The listing builds one solid part. Answer for the finished solid, in the listing's coordinates (mm). Face numbers are marked on the shaded views. Give positions to 0.01 mm unless a question says otherwise; leave off trailing zeros. Order: outer loops, then holes, each group sorted by start corner. A loop starts at its lowest first (then second) coordinate and runs counter-clockwise, first axis right, second up. Notation, with made-up numbers: M -25.75,-12.75 L -9.75,-12.75 A16 cw -9.75,-3.75 Z; hole C 59,73 d2. An arc over 180 degrees is marked long. Answer as a JSON object with one key per item and string values. Group by question number.
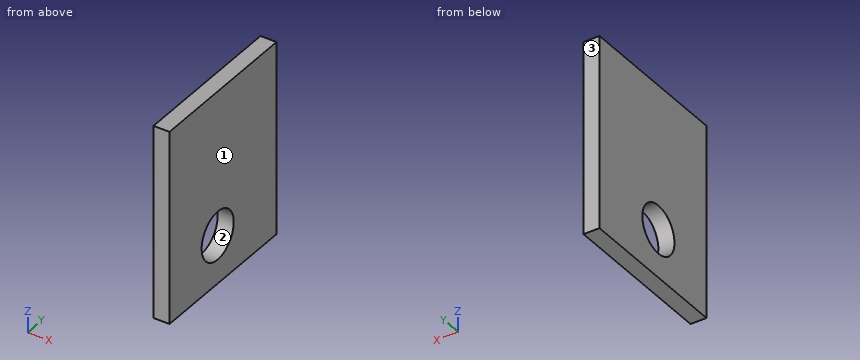
```python
from build123d import *

# Parameters (mm, degrees)
CYLINDER3125_R               = 1.5
CYLINDER3125_DEPTH           = 12
CYLINDER3127_R               = 1.5
CYLINDER3127_DEPTH           = 4
BOX1135_W                    = 6
BOX1135_H                    = 6
BOX1135_DEPTH                = 2
COMPOUND1374_PLACEMENT_ANGLE = 90
BOX1136_W                    = 1
BOX1136_H                    = 10
BOX1136_DEPTH                = 12


with BuildPart() as obj1:
    # Cylinder3125 → Cylinder3125 (new body)
    with BuildSketch(Plane(origin=(1, 14, 6), x_dir=(1, 0, 0), z_dir=(0, 0, 1))):
        Circle(CYLINDER3125_R)
    extrude(amount=CYLINDER3125_DEPTH)


with BuildPart() as obj2:
    # Cylinder3127 → Cylinder3127 (new body)
    with BuildSketch(Plane(origin=(1, 14, -0.1), x_dir=(1, 0, 0), z_dir=(0, 0, 1))):
        Circle(CYLINDER3127_R)
    extrude(amount=CYLINDER3127_DEPTH)


with BuildPart() as compound1374:
    # Box1135 → Box1135 (new body)
    with BuildSketch(Plane(origin=(-2, 11, 4), x_dir=(1, 0, 0), z_dir=(0, 0, 1))):
        with Locations((3, 3)):
            Rectangle(BOX1135_W, BOX1135_H)
    extrude(amount=BOX1135_DEPTH)

    # Compound1374: union obj1, obj2
    add(obj1.part)
    add(obj2.part)


with BuildPart() as compound1374_1:
    # Compound1374 placement: moved
    add(compound1374.part.moved(Location((6, -14, 2))).rotate(Axis((6, -14, 2), (0, 1, 0)), COMPOUND1374_PLACEMENT_ANGLE))


with BuildPart() as cut1267:
    # Box1136 → Box1136 (new body)
    with BuildSketch(Plane(origin=(21.4, -4.5, -2), x_dir=(1, 0, 0), z_dir=(0, 0, 1))):
        with Locations((0.5, 5)):
            Rectangle(BOX1136_W, BOX1136_H)
    extrude(amount=BOX1136_DEPTH)

    # Cut1267: cut Compound1374
    add(compound1374_1.part, mode=Mode.SUBTRACT)


with BuildPart() as cut1267_1:
    # Cut1267 placement: moved
    add(cut1267.part.moved(Location((0.2, 0, 0))))


solid = cut1267_1.part
```
Item 1: Determine the mould class of the marked faces 1, 2 and 3 for opening direction Y: released by +Y, released by -Y, zero draft, split by the parting line, or undercut.
Item 2: Section A-A (y = 0) is taken. Determine the outline of the cut face in (x, z), and give its area (3 significant figures).
Item 3: Section B-B (x = 22.15) is taken. Determine the outline of the cut face in (y, z).
Item 4: Consider probe 1 along Z at (x, y) = (22.05, 0); probe 2 along Y at (x, z) = (22.1, 1); probe 3 along Y at (x, z) = (21.7, 1.5). Determine where each line is inside the solid, lowest interval first. Write a range as from..to.
Item 5: Section C-C (z = 1) is taken. Determine the outline of the cut face in (x, y).
Values found:
{
 "1": {"face 1": "zero draft", "face 2": "undercut", "face 3": "released by +Y"},
 "2": {"outline": "M 21.6,-2 L 22.6,-2 L 22.6,-0.5 L 21.6,-0.5 Z; M 21.6,2.5 L 22.6,2.5 L 22.6,10 L 21.6,10 Z", "area": "9.00 mm^2"},
 "3": {"outline": "M -4.5,-2 L 5.5,-2 L 5.5,10 L -4.5,10 Z; hole C 0,1 d3"},
 "4": {"probe 1": "z = -2..-0.5, 2.5..10", "probe 2": "y = -4.5..-1.5, 1.5..5.5", "probe 3": "y = -4.5..-1.41, 1.41..5.5"},
 "5": {"outline": "M 21.6,-4.5 L 22.6,-4.5 L 22.6,-1.5 L 21.6,-1.5 Z; M 21.6,1.5 L 22.6,1.5 L 22.6,5.5 L 21.6,5.5 Z"}
}
